Read the model definition and answer for the solid it produces. Units are mm, in the model's axes. A direction names the side the tool comes from. Give positions to 0.01 mm unless a question says otherwise; leave off trailing zeros. Order: outer loops, then holes, each group sorted by start corner. A loop starts at its lowest first (then second) coordinate and runs counter-clockwise, first axis right, second up.
Item 1: A cutting plane is placed at D-D (x = -23.5). Write down the section's boundary in (y, z), plus the area to 3 significant figures.
Item 2: Which of the six approach directions +Z, -Z, +X, -X, +Y, -Y give full straight-line access (tool end or side, diameter ignored) to faces 1 (the face through (21.4, 9.8, 41.1)), 2 (the face through (0, 0, 0)), 3 (the face through (-17, -0.658, 40))?
Item 3: Find the intervals of material crossed by line 1 along X through (y, z) = (4.5, 41); line 2 along X through (y, z) = (13.5, 46); line 3 along Z through (x, y) = (-21.5, 5.5), in increasing order.
Item 4: A cutting plane is placed at B-B (y = 10). Write down the section's boundary in (x, z), plus the area to 3 significant figures.
Item 5: A cutting plane is placed at C-C (z = 44.5). Write down the section's boundary in (x, y), plus the area to 3 significant figures.
Item 6: Given pin 1 Ø9.5 at (x, z) = (-11, 40) entering from +Y; pin 2 Ø1 at (y, z) = (4.5, 32.5) entering from -X; pin 3 Ø15.5 at (y, z) = (14, 37) entering from -X; pin 4 Ø10 at (x, y) = (-20, 6.5) entering from +Z, each flat-ended and moving along its own axis, determine where each tip first touches the part or whether it passes through.
Item 7: A cutting plane is placed at A-A (x = 21.5). Write down the section's boundary in (y, z), plus the area to 3 significant figures.
Autodesk Inventor part; units mm, degrees
ref_plane "YZ Plane" through (0, 0, 0) normal (1, 0, 0) x (0, 1, 0)
ref_plane "XZ Plane" through (0, 0, 0) normal (0, 1, 0) x (-1, 0, 0)
ref_plane "XY Plane" through (0, 0, 0) normal (0, 0, 1) x (1, 0, 0)
sketch "스케치1" plane through (0, 0, 0) normal (0, 0, 1) x (1, 0, 0)
  line L0 (28.7473, -19.3425) -> (-28.7473, -19.3425)
  line L1 (-28.7473, -19.3425) -> (-28.7473, 19.3425)
  line L2 (-28.7473, 19.3425) -> (28.7473, 19.3425)
  line L3 (28.7473, 19.3425) -> (28.7473, -19.3425)
  line L4 (28.7473, -19.3425) -> (-28.7473, 19.3425) construction
  line L5 (-28.7473, -19.3425) -> (28.7473, 19.3425) construction
  point P0 (0, 0)
extrude "돌출1" add sketch "스케치1" along normal blind 50
sketch "스케치2" plane through (-28.7473, 19.3425, 0) normal (0, 1, 0) x (1, 0, 0)
  line L0 (0, -50) -> (57.4945, -50)
  line L1 (0, -50) -> (24.4372, -50)
  line L2 (24.4372, -50) -> (24.4372, -30.5624)
  line L3 (24.4372, -30.5624) -> (0, -30.5624)
  line L4 (0, -30.5624) -> (0, -50)
  point P0 (28.7473, 0)
extrude "돌출2" cut sketch "스케치2" against normal blind 20
sketch "스케치3" plane through (28.7473, -19.3425, 0) normal (1, 0, 0) x (0, 0, -1)
  point P0 (0, 19.3425)
sketch "스케치4" plane through (28.7473, -19.3425, 0) normal (1, 0, 0) x (0, 0, -1)
  line L0 (0, 38.685) -> (-50, 38.685)
  line L1 (-32.4307, 38.685) -> (-50, 19.3425)
  line L2 (-50, 0) -> (-50, 38.685)
  point P0 (0, 19.3425)
extrude "돌출3" cut sketch "스케치4" against normal blind 15
properties part number "240503_3Dsketch05"
Response values:
1. outline: (-19.34, 0) - (19.34, 0) - (19.34, 30.56) - (-0.66, 30.56) - (-0.66, 50) - (-19.34, 50) - close
1. area: 1,550 mm2
2. face 1: +Z, +X, +Y
2. face 2: -Z, +X, -X, +Y, -Y
2. face 3: +Z, -X, +Y
3. line 1: x = -4.31 to 28.75
3. line 2: x = -4.31 to 13.75
3. line 3: z = 0 to 30.56
4. outline: (-28.75, 0) - (28.75, 0) - (28.75, 40.92) - (13.75, 40.92) - (13.75, 50) - (-4.31, 50) - (-4.31, 30.56) - (-28.75, 30.56) - close
4. area: 2,260 mm2
5. outline: (-28.75, -19.34) - (28.75, -19.34) - (28.75, 6.06) - (13.75, 6.06) - (13.75, 19.34) - (-4.31, 19.34) - (-4.31, -0.66) - (-28.75, -0.66) - close
5. area: 1,540 mm2
6. pin 1: stops at y = -0.66
6. pin 2: stops at x = -4.31
6. pin 3: stops at x = -28.75
6. pin 4: stops at z = 30.56
7. outline: (-19.34, 0) - (19.34, 0) - (19.34, 32.43) - (0, 50) - (-19.34, 50) - close
7. area: 1,760 mm2
